from build123d import *
from OCP.BRepFilletAPI import BRepFilletAPI_MakeFillet

# Parameters (mm, degrees)
SKETCH1_W               = 57
SKETCH1_H               = 122
BOSS_EXTRUDE1_DEPTH     = 6.6
FILLET1_R               = 4.5
SKETCH2_R               = 2.5
CUT_EXTRUDE1_DEPTH      = 68.652124874
SKETCH3_R               = 3.75
CUT_EXTRUDE2_DEPTH      = 4.1
MIRROR3_COPY_1_SKETCH_R = 2.5
MIRROR3_COPY_1_DEPTH    = 68.652124874
MIRROR3_COPY_2_SKETCH_R = 3.75
MIRROR3_COPY_2_DEPTH    = 4.1
CUT_EXTRUDE3_DEPTH      = 4.1
FILLET2_R               = 10
FILLET3_R               = 2
FILLET2_OF_MIRROR4_R    = 10
FILLET3_OF_MIRROR4_R    = 2
MIRROR5_START           = 2.5
MIRROR5_DEPTH           = 4.1
FILLET4_R1              = 2
FILLET4_R2              = 6


with BuildPart() as part:
    # Sketch1 → Boss-Extrude1 (new body)
    with BuildSketch(Plane(origin=(0, 0, 0), x_dir=(1, 0, 0), z_dir=(0, 1, 0))):
        Rectangle(SKETCH1_W, SKETCH1_H)
    extrude(amount=BOSS_EXTRUDE1_DEPTH)

    # Fillet1
    fillet1_edges = [part.edges().sort_by_distance(p)[0] for p in [
        (28.5, 3.3, 61),
        (-28.5, 3.3, 61),
        (-28.5, 3.3, -61),
        (28.5, 3.3, -61),
    ]]
    fillet(fillet1_edges, radius=FILLET1_R)

    # Sketch2 → Cut-Extrude1 (cut, through all)
    with BuildSketch(Plane(origin=(0, 6.6, 0), x_dir=(1, 0, 0), z_dir=(0, 1, 0))):
        with Locations(Location((20.5, 53, 0), (0, 0, 270))):
            Circle(SKETCH2_R)
    cut_extrude1 = extrude(amount=-CUT_EXTRUDE1_DEPTH, mode=Mode.SUBTRACT)

    # Sketch3 → Cut-Extrude2 (cut)
    with BuildSketch(Plane(origin=(0, 6.6, 0), x_dir=(1, 0, 0), z_dir=(0, 1, 0))):
        with Locations(Location((20.5, 53, 0), (0, 0, 270))):
            Circle(SKETCH3_R)
    cut_extrude2 = extrude(amount=-CUT_EXTRUDE2_DEPTH, mode=Mode.SUBTRACT)

    # Mirror1: Cut-Extrude1, Cut-Extrude2 across plane
    add(cut_extrude1.mirror(Plane(origin=(0, 0, 0), x_dir=(0, 0, 1), z_dir=(1, 0, 0))), mode=Mode.SUBTRACT)
    add(cut_extrude2.mirror(Plane(origin=(0, 0, 0), x_dir=(0, 0, 1), z_dir=(1, 0, 0))), mode=Mode.SUBTRACT)

    # Mirror3: Cut-Extrude1, Cut-Extrude2 across plane
    add(cut_extrude1.mirror(Plane.XY), mode=Mode.SUBTRACT)
    add(cut_extrude2.mirror(Plane.XY), mode=Mode.SUBTRACT)

    # Mirror3 copy 1 sketch → Mirror3 copy 1 (cut, through all)
    with BuildSketch(Plane(origin=(0, 6.6, 0), x_dir=(-1, 0, 0), z_dir=(0, 1, 0))):
        with Locations(Location((20.5, 53, 0), (0, 0, 270))):
            Circle(MIRROR3_COPY_1_SKETCH_R)
    extrude(amount=-MIRROR3_COPY_1_DEPTH, mode=Mode.SUBTRACT)

    # Mirror3 copy 2 sketch → Mirror3 copy 2 (cut)
    with BuildSketch(Plane(origin=(0, 6.6, 0), x_dir=(-1, 0, 0), z_dir=(0, 1, 0))):
        with Locations(Location((20.5, 53, 0), (0, 0, 270))):
            Circle(MIRROR3_COPY_2_SKETCH_R)
    extrude(amount=-MIRROR3_COPY_2_DEPTH, mode=Mode.SUBTRACT)

    # Sketch4 → Cut-Extrude3 (cut)
    with BuildSketch(Plane(origin=(0, 6.6, 0), x_dir=(1, 0, 0), z_dir=(0, 1, 0))):
        with BuildLine():
            Line((0, 57), (0, 4.825290504))
            Line((0, 4.825290504), (18.422458297, 45.274469567))
            ThreePointArc((18.422458297, 45.274469567), (13.107579799, 49.941875809), (13.57179677, 57))
            Line((13.57179677, 57), (0, 57))
        make_face()
        with BuildLine():
            Line((24.5, 0), (24.5, 46.07179677))
            ThreePointArc((24.5, 46.07179677), (23.697246566, 45.666677806), (22.854101194, 45.354203274))
            Line((22.854101194, 45.354203274), (2.197664208, 0))
            Line((2.197664208, 0), (24.5, 0))
        make_face()
    cut_extrude3 = extrude(amount=-CUT_EXTRUDE3_DEPTH, mode=Mode.SUBTRACT)

    # Fillet2
    # the kernel refuses this fillet: 10 mm, written as the material it adds along each edge
    with BuildSketch(Plane(origin=(22.854101194, 6.6, -45.354203274), x_dir=(0.9166652742214988, 0, -0.3996558207213108), z_dir=(0, -1, 0))) as fillet2_piece_1:
        with BuildLine():
            CenterArc((4.145887895, 9.719866853), FILLET2_R, 228.043415152, 28.362844717)
            Line((-2.539785162, 2.28335048), (-2.673498623, 2.134620152))
            Line((-2.673498623, 2.134620152), (-0.133713461, -0.148730327))
            Line((-0.133713461, -0.148730327), (0.022444109, -0.198736665))
            ThreePointArc((0.022444109, -0.198736665), (0.897764349, -0.149466597), (1.748521514, -0.194397337))
            Line((1.748521514, -0.194397337), (1.795528698, 0))
        make_face()
    extrude(amount=4.1)
    with BuildSketch(Plane(origin=(18.422458297, 6.6, -45.274469567), x_dir=(-0.41448281678671633, 0, 0.9100571380899934), z_dir=(0, -1, 0))) as fillet2_piece_2:
        with BuildLine():
            CenterArc((7.872374254, 10), FILLET2_R, 208.861826981, 61.138173019)
            Line((-0.885488916, 5.173009977), (-1.06064618, 5.076470177))
            ThreePointArc((-1.06064618, 5.076470177), (-0.203601176, 2.627440291), (-0.197294486, 0.032785449))
            Line((-0.197294486, 0.032785449), (0, -0.2))
            Line((0, -0.2), (7.872374254, -0.2))
            Line((7.872374254, -0.2), (7.872374254, 0))
        make_face()
    extrude(amount=4.1)

    # Fillet3
    # the kernel refuses this fillet: 2 mm, written as the material it adds along each edge
    with BuildSketch(Plane(origin=(13.57179677, 6.6, -57), x_dir=(-0.3545926272331019, 0, 0.9350208921259068), z_dir=(0, -1, 0))) as fillet3_piece_1:
        with BuildLine():
            CenterArc((2.887636012, 1.974096319), FILLET3_R, 159.231520484, 101.536959033)
            Line((1.017594228, 2.683281573), (0, 0))
            ThreePointArc((0, 0), (1.283393783, 0.103614726), (2.566787566, 0))
        make_face()
    extrude(amount=4.1)
    with BuildSketch(Plane(origin=(24.5, 6.6, -46.07179677), x_dir=(-0.5710655658719064, 0, 0.8209044520986588), z_dir=(0, -1, 0))) as fillet3_piece_2:
        with BuildLine():
            CenterArc((6.330546511, -1.967533641), FILLET3_R, 79.662186843, 155.513248783)
            Line((5.18841538, -3.609342545), (5.074202266, -3.773523436))
            Line((5.074202266, -3.773523436), (-0.114213113, -0.16418089))
            Line((-0.114213113, -0.16418089), (-0.061886493, 0.190184284))
            ThreePointArc((-0.061886493, 0.190184284), (4.924730005, 0.525207358), (6.725339822, 0.196753364))
            Line((6.725339822, 0.196753364), (6.689449521, 0))
        make_face()
    extrude(amount=4.1)

    # Mirror4: Cut-Extrude3 across plane
    add(cut_extrude3.mirror(Plane(origin=(0, 0, 0), x_dir=(0, 0, 1), z_dir=(1, 0, 0))), mode=Mode.SUBTRACT)

    # Fillet2 of Mirror4
    # the kernel refuses this fillet: 10 mm, written as the material it adds along each edge
    with BuildSketch(Plane(origin=(-22.854101194, 6.6, -45.354203274), x_dir=(0.4144828167867165, 0, 0.9100571380899934), z_dir=(0, -1, 0))) as fillet2_of_mirror4_piece_1:
        with BuildLine():
            CenterArc((3.415288872, 10), FILLET2_OF_MIRROR4_R, 241.637155283, 28.362844717)
            Line((-1.335247856, 1.200431784), (-1.43025859, 1.024440419))
            ThreePointArc((-1.43025859, 1.024440419), (-0.767552408, 0.489064812), (-0.149559435, -0.132785449))
            Line((-0.149559435, -0.132785449), (0, -0.2))
            Line((0, -0.2), (3.415288872, -0.2))
            Line((3.415288872, -0.2), (3.415288872, 0))
        make_face()
    extrude(amount=4.1)
    with BuildSketch(Plane(origin=(-18.422458297, 6.6, -45.274469567), x_dir=(0.8270785739825625, 0, -0.5620863211811608), z_dir=(0, -1, 0))) as fillet2_of_mirror4_piece_2:
        with BuildLine():
            CenterArc((8.528405442, 9.446723083), FILLET2_OF_MIRROR4_R, 189.713452681, 61.138173019)
            Line((-1.328233375, 7.759514966), (-1.525366151, 7.725770803))
            Line((-1.525366151, 7.725770803), (-0.197132776, -0.033744162))
            Line((-0.197132776, -0.033744162), (0.065603119, -0.188934462))
            ThreePointArc((0.065603119, -0.188934462), (2.624124751, 0.242621533), (5.182646384, -0.188934462))
            Line((5.182646384, -0.188934462), (5.248249503, 0))
        make_face()
    extrude(amount=4.1)

    # Fillet3 of Mirror4
    # the kernel refuses this fillet: 2 mm, written as the material it adds along each edge
    with BuildSketch(Plane(origin=(-13.57179677, 6.6, -57), x_dir=(0.35459262723310125, 0, 0.935020892125907), z_dir=(0, -1, 0))) as fillet3_of_mirror4_piece_1:
        with BuildLine():
            CenterArc((2.887636012, -1.974096319), FILLET3_OF_MIRROR4_R, 99.231520484, 101.536959033)
            Line((1.017594228, -2.683281573), (0, 0))
            ThreePointArc((0, 0), (1.283393783, -0.103614726), (2.566787566, 0))
        make_face()
    extrude(amount=4.1)
    with BuildSketch(Plane(origin=(-24.5, 6.6, -46.07179677), x_dir=(0.5710655658719064, 0, 0.8209044520986588), z_dir=(0, -1, 0))) as fillet3_of_mirror4_piece_2:
        with BuildLine():
            CenterArc((6.330546511, 1.967533641), FILLET3_OF_MIRROR4_R, 124.824564374, 155.513248783)
            Line((5.18841538, 3.609342545), (5.074202266, 3.773523436))
            Line((5.074202266, 3.773523436), (-0.114213113, 0.16418089))
            Line((-0.114213113, 0.16418089), (-0.061886493, -0.190184284))
            ThreePointArc((-0.061886493, -0.190184284), (4.924730005, -0.525207358), (6.725339822, -0.196753364))
            Line((6.725339822, -0.196753364), (6.689449521, 0))
        make_face()
    extrude(amount=4.1)

    # Mirror5: read off the stored shape, not the designer's step
    # Mirror5 outline → Mirror5 (cut)
    with BuildSketch(Plane(origin=(0, 0, 0), x_dir=(1, 0, 0), z_dir=(0, 1, 0)).offset(MIRROR5_START)):
        with BuildLine():
            Line((-20.679885724, -40.580397876), (-2.197664208, 0))
            Line((-2.197664208, 0), (-24.5, 0))
            Line((-24.5, 0), (-24.5, -39.751432242))
            ThreePointArc((-24.5, -39.751432242), (-22.924129372, -41.705943505), (-20.679885724, -40.580397876))
        make_face()
        with BuildLine():
            ThreePointArc((20.679885724, -40.580397876), (22.924129372, -41.705943505), (24.5, -39.751432242))
            Line((24.5, -39.751432242), (24.5, 0))
            Line((24.5, 0), (2.197664208, 0))
            Line((2.197664208, 0), (20.679885724, -40.580397876))
        make_face()
        with BuildLine():
            Line((15.159494442, -38.110159183), (0, -4.825290504))
            Line((0, -4.825290504), (-15.159494442, -38.110159183))
            ThreePointArc((-15.159494442, -38.110159183), (-16.002629649, -43.314562397), (-14.081743582, -48.224438823))
            ThreePointArc((-14.081743582, -48.224438823), (-12.69136541, -51.260682364), (-12.661632823, -54.6))
            ThreePointArc((-12.661632823, -54.6), (-12.251234367, -56.264911064), (-10.702041029, -57))
            Line((-10.702041029, -57), (10.702041029, -57))
            ThreePointArc((10.702041029, -57), (12.251234367, -56.264911064), (12.661632823, -54.6))
            ThreePointArc((12.661632823, -54.6), (12.69136541, -51.260682364), (14.081743582, -48.224438823))
            ThreePointArc((14.081743582, -48.224438823), (16.002629649, -43.314562397), (15.159494442, -38.110159183))
        make_face()
    extrude(amount=MIRROR5_DEPTH, mode=Mode.SUBTRACT)

    # Fillet4: one fillet with a radius per group of edges: ONE call of the kernel's fillet builder (fillet() takes one radius for all edges)
    fillet4_edges_1 = [part.edges().sort_by_distance(p)[0] for p in [
        (0, 4.55, -4.825290504),
        (0, 4.55, 4.825290504),
    ]]
    fillet4_edges_2 = [part.edges().sort_by_distance(p)[0] for p in [
        (-2.197664208, 4.55, 0),
        (2.197664208, 4.55, 0),
    ]]
    fillet4 = BRepFilletAPI_MakeFillet(part.part.solid().wrapped)
    for e in fillet4_edges_1:
        fillet4.Add(FILLET4_R1, e.wrapped)
    for e in fillet4_edges_2:
        fillet4.Add(FILLET4_R2, e.wrapped)
    add(Compound.cast(fillet4.Shape()), mode=Mode.REPLACE)


solid = part.part
Geometry: final body of the model. Coordinates: model frame, mm. A direction names the side the tool comes from. Coordinates: 2 decimals unless noted, no trailing zeros. Loops run counter-clockwise (first coordinate to the right, second up) from the corner with the lowest first, then second, coordinate; pieces in that order, holes last. Notation, with made-up numbers: M 73.5,-16.75 L 91.5,-16.75 A19 ccw 91.5,3.25 Z; hole C 55,3 d11. An arc over 180 degrees is marked long. One line per item, written item: value. Start each with the question number.
1) Cut plane B-B (z = 1). Return loops of the section in (x, y), then the cut area to 3 significant figures.
2) Cut plane C-C (y = 5). Count the separate pieces of the cut face and the enclosed holes in it, then the cut area to 3 significant figures.
3) Pin query (flat end, axial travel): P1, Ø12, axis at x = 6, z = 41, coming from the +Y side; P2, Ø4.5, axis at x = 20.5, z = 53, coming from the -Y side. Return the tip coordinate at first contact, or that it passes through.
4) Draft query along Z for faces 3 (the flat face through (-8.396, 4.521, 23.261)), 4 (the flat face through (28.5, 3, 1)), 5 (the flat face through (0, 3, 61)). Return one class per face: released by +Z, released by -Z, zero draft, split by the parting line, or undercut.
5) Material intervals for L1, parallel to X at y = 1.65, z = 53; L2, parallel to Z at x = 15, y = 5.5; L3, parallel to Z at x = -20.5, y = 4.1, sorted ascending. Write a range as from..to.
6) Reachability of faces 1 (the cylindrical face through (-27.217, 3.346, -59.647)), 2 (the flat face through (18, 2.5, -52)) from +Z, -Z, +X, -X, +Y, -Y: full face, straight path, thin tool, end or side. Return the list, or none.
7) Cut plane A-A (z = 53). Return loops of the section in (x, y).
8) Cut plane D-D (z = -22.5). Return loops of the section in (x, y), then the cut area to 3 significant figures.
Evaluation:
1. outline: M -28.5,0 L 28.5,0 L 28.5,6.6 L 24.5,6.6 L 24.5,2.5 L 2.87,2.5 L 2.87,6.6 L -2.87,6.6 L -2.87,2.5 L -24.5,2.5 L -24.5,6.6 L -28.5,6.6 Z
1. area: 199 mm^2
2. separate pieces: 1
2. enclosed holes: 8
2. area: 2,550 mm^2
3. P1: y = 2.5
3. P2: through
4. face 3: undercut
4. face 4: zero draft
4. face 5: released by +Z
5. L1: -28.5..-23, -18..18, 23..28.5
5. L2: -61..-46.73, -37.76..-28.11, 28.11..37.76, 46.73..61
5. L3: -61..-56.75, -49.25..-40.19, 40.19..49.25, 56.75..61
6. face 1: -Z, -X, +Y, -Y
6. face 2: +Y
7. outline: M -28.5,0 L -23,0 L -23,2.5 L -24.25,2.5 L -24.25,6.6 L -28.5,6.6 Z; M -18,0 L 18,0 L 18,2.5 L 16.75,2.5 L 16.75,6.6 L 12.5,6.6 L 12.5,2.5 L -12.5,2.5 L -12.5,6.6 L -16.75,6.6 L -16.75,2.5 L -18,2.5 Z; M 23,0 L 28.5,0 L 28.5,6.6 L 24.25,6.6 L 24.25,2.5 L 23,2.5 Z
8. outline: M -28.5,0 L 28.5,0 L 28.5,6.6 L 24.5,6.6 L 24.5,2.5 L 12.45,2.5 L 12.45,6.6 L 8.05,6.6 L 8.05,2.5 L -8.05,2.5 L -8.05,6.6 L -12.45,6.6 L -12.45,2.5 L -24.5,2.5 L -24.5,6.6 L -28.5,6.6 Z
8. area: 211 mm^2
